from build123d import *

# Parameters (mm, degrees)
F1_DEPTH = 25
F4_DEPTH = 30.001
F5_DEPTH = 30.001


with BuildPart() as f1:
    # F0 (on Top) → F1 (new body)
    with BuildSketch(Plane.XY):
        Polygon((0, 0), (-15, 15), (-15, -15), align=None)
        Polygon((15, 15), (-15, 15), (0, 0), align=None)
        Polygon((15, -15), (15, 15), (0, 0), align=None)
        Polygon((0, 0), (-15, -15), (15, -15), align=None)
    extrude(amount=F1_DEPTH)

    # F3 (on face) → F4 (cut, through all)
    with BuildSketch(Plane.XZ.offset(15)):
        Polygon((-15, 25), (-15, 5), (0, 25), align=None)
        Polygon((0, 25), (15, 5), (15, 25), align=None)
    extrude(amount=-F4_DEPTH, mode=Mode.SUBTRACT)

    # F2 (on face) → F5 (cut, through all)
    with BuildSketch(Plane.YZ.offset(15)):
        Polygon((-15, 25), (-15, 5), (0, 25), align=None)
        Polygon((0, 25), (15, 5), (15, 25), align=None)
    extrude(amount=-F5_DEPTH, mode=Mode.SUBTRACT)

    # F6 (on Front) → F7 (revolve)
    with BuildSketch(Plane.XZ):
        with BuildLine():
            ThreePointArc((0, 10), (5.3033008589, 12.1966991411), (7.5, 17.5))
            ThreePointArc((7.5, 17.5), (5.3033008589, 22.8033008589), (0, 25))
            Line((0, 25), (0, 10))
        make_face()
    revolve(axis=Axis((0, 0, 17.5), (0, 0, 1)))


solid = f1.part
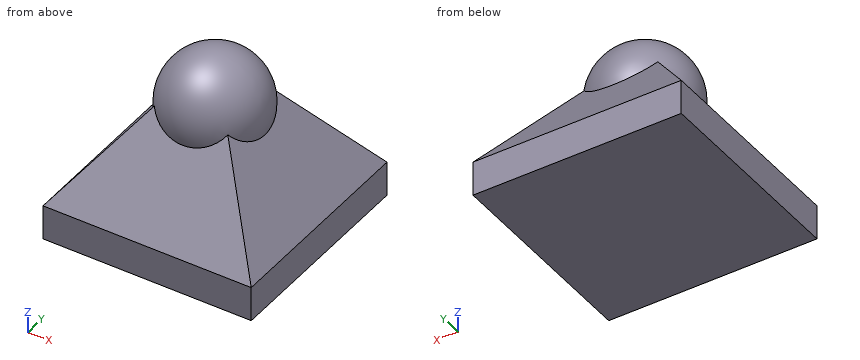
Build history of the part. All positions in model axes, mm. Round coordinates to 2 decimals unless told otherwise and drop trailing zeros. Write each loop counter-clockwise with the first axis right and the second up, starting at its lowest first coordinate (ties: lowest second). Pieces come first, ordered by that corner, then holes. Notation, with made-up numbers: (9.25, -19.5) - (65.25, -19.5) arc R30 ccw to (65.25, 12.5) - close; hole circle Ø11 at (61, 63). An arc over 180 degrees is marked (long way). One line per question, with ' | ' between items.
1. Band-saw the part on C-C, the plane y = 9.5. Write the cut outline in (x, z), and give its area (3 significant figures).
Results are:
outline: (-15, 0) - (15, 0) - (15, 5) - (9.5, 12.33) - (-9.5, 12.33) - (-15, 5) - close | area: 330 mm^2
2. Drill centre lines: line 1 along Z through (x, y) = (-3.75, 7.5); line 2 along Y through (x, z) = (1, 20); line 3 along Y through (x, z) = (11.75, 9.25). Where is each one in solid material? Low to high. Write a range as from..to.
Results are:
line 1: 0..15 | line 2: -7..7 | line 3: -11.81..11.81
3. Drop flat-ended pins along their axis: pin 1 Ø12 at (x, y) = (5, 10) entering from +Z; pin 2 Ø10 at (x, y) = (-9.5, -3.5) entering from +Z; pin 3 Ø10 at (y, z) = (6.5, 17.5) entering from +X (3 decimals). Give the stop position or say it passes through.
Results are:
pin 1: z = 22.92 | pin 2: z = 22.98 | pin 3: x = 9.375
4. Band-saw the part on B-B, the plane z = 16. Write the cut outline in (x, y), and give its area (3 significant figures).
Results are:
outline: (-6.75, -6.75) - (-2.9, -6.75) arc R7.35 ccw to (2.9, -6.75) - (6.75, -6.75) - (6.75, -2.9) arc R7.35 ccw to (6.75, 2.9) - (6.75, 6.75) - (2.9, 6.75) arc R7.35 ccw to (-2.9, 6.75) - (-6.75, 6.75) - (-6.75, 2.9) arc R7.35 ccw to (-6.75, -2.9) - close | area: 192 mm^2
5. Band-saw the part on D-D, the plane x = -6.25. Write the cut outline in (y, z), and give its area (3 significant figures).
Results are:
outline: (-15, 0) - (15, 0) - (15, 5) - (6.25, 16.67) - (4.06, 16.67) arc R4.15 ccw (long way) to (-4.06, 16.67) - (-6.25, 16.67) - (-15, 5) - close | area: 432 mm^2
6. Band-saw the part on A-A, the plane x = 12. Write the cut outline in (y, z), and give its area (3 significant figures).
Results are:
outline: (-15, 0) - (15, 0) - (15, 5) - (12, 9) - (-12, 9) - (-15, 5) - close | area: 258 mm^2
